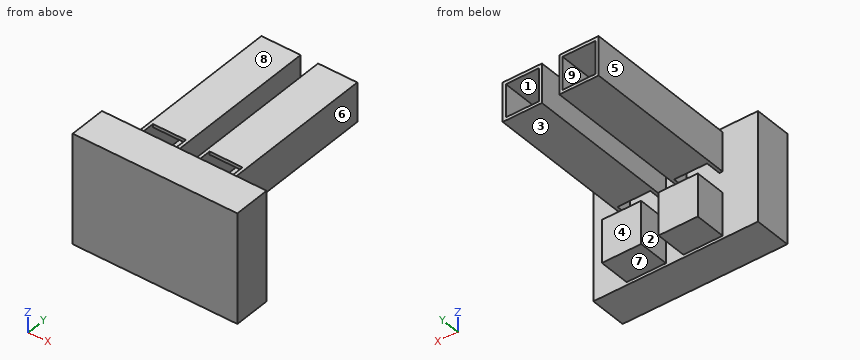
```python
from build123d import *

# Parameters (mm, degrees)
SKETCH1_W           = 266.7
SKETCH1_H           = 177.8
BOSS_EXTRUDE1_DEPTH = 59.944
SKETCH2_W           = 63.5
SKETCH2_H           = 63.5
SKETCH2_W_2         = 53.34
SKETCH2_H_2         = 53.34
BOSS_EXTRUDE2_DEPTH = 254
SKETCH3_W           = 53.34
SKETCH3_H           = 25.4
CUT_EXTRUDE1_DEPTH  = 254
SKETCH4_W           = 63.5
SKETCH4_H           = 69.373154479
BOSS_EXTRUDE3_DEPTH = 50.8
SKETCH5_R           = 6.35
CUT_EXTRUDE2_DEPTH  = 50.8


with BuildPart() as part:
    # Sketch1 → Boss-Extrude1 (new body)
    with BuildSketch(Plane(origin=(0, 0, 0), x_dir=(1, 0, 0), z_dir=(0, 1, 0))):
        with Locations((133.35, 88.9)):
            Rectangle(SKETCH1_W, SKETCH1_H)
    extrude(amount=BOSS_EXTRUDE1_DEPTH)

    # Sketch2 → Boss-Extrude2 (add)
    with BuildSketch(Plane(origin=(0, 59.944, 0), x_dir=(1, 0, 0), z_dir=(0, 1, 0))):
        with Locations((180.927983049, 38.1)):
            Rectangle(SKETCH2_W, SKETCH2_H)
        with Locations((180.927983049, 38.260329554)):
            Rectangle(SKETCH2_W_2, SKETCH2_H_2, mode=Mode.SUBTRACT)
        with Locations((89.140378802, 38.1)):
            Rectangle(SKETCH2_W, SKETCH2_H)
        with Locations((89.140378802, 38.260329554)):
            Rectangle(SKETCH2_W_2, SKETCH2_H_2, mode=Mode.SUBTRACT)
    extrude(amount=BOSS_EXTRUDE2_DEPTH)

    # Sketch3 → Cut-Extrude1 (cut)
    with BuildSketch(Plane.XY.offset(-6.35)):
        with Locations((89.140378802, 72.644)):
            Rectangle(SKETCH3_W, SKETCH3_H)
        with Locations((180.927983049, 72.644)):
            Rectangle(SKETCH3_W, SKETCH3_H)
    extrude(amount=-CUT_EXTRUDE1_DEPTH, mode=Mode.SUBTRACT)

    # Sketch4 → Boss-Extrude3 (add)
    with BuildSketch(Plane(origin=(0, 59.944, 0), x_dir=(1, 0, 0), z_dir=(0, 1, 0))):
        with Locations((89.140378802, 138.306511279)):
            Rectangle(SKETCH4_W, SKETCH4_H)
        with Locations((180.927983049, 138.306511279)):
            Rectangle(SKETCH4_W, SKETCH4_H)
    extrude(amount=BOSS_EXTRUDE3_DEPTH)

    # Sketch5 → Cut-Extrude2 (cut)
    with BuildSketch(Plane.XY.offset(-103.619934039)):
        with Locations((180.927983049, 72.644)):
            Circle(SKETCH5_R)
        with Locations((89.140378802, 72.644)):
            Circle(SKETCH5_R)
    extrude(amount=-CUT_EXTRUDE2_DEPTH, mode=Mode.SUBTRACT)


solid = part.part
```
Build history of the part. All positions in model axes, mm. Face numbers are marked on the shaded views. A direction names the side the tool comes from. Coordinates: 2 decimals unless noted, no trailing zeros. Order: outer loops, then holes, each group sorted by start corner. A loop starts at its lowest first (then second) coordinate and runs counter-clockwise, first axis right, second up. Notation, with made-up numbers: (-3.75, -15.5) -> (23.25, -15.5) arc R31 cw to (23.25, 22.5) -> close; hole circle Ø1 at (-22, -37). An arc over 180 degrees is marked (long way). Answer in a Markdown table with one row per item. Add a question column.
Q1. Band-saw the part on B-B, the plane x = 107. List the corners of the cut face in (y, z).
Q2. Band-saw the part on A-A, the plane y = 93.5. List the corners of the cut face in (x, z).
Q3. Wall check: line 1 along X through (y, z) = (98, -40); line 2 along Z through (x, y) = (202, 101.5); line 3 along Z through (x, y) = (172.5, 221). Give the ranges that are in metal, low to high. Write a range as [from, to].
Q4. Which spindle directions (+Z, -Z, +X, -X, +Y, -Y) get a long thin tool onto all of the face, cutting with end or side? Do the marked faces 1, 2, 3, 4 and 5. Say none if no direction does.
Q5. Drop flat-ended pins along their axis: pin 1 (10 mm diameter, centred on x = 180.93, y = 72.64, fed in from +Z); pin 2 (1 mm diameter, centred on x = 165, y = 110, fed in from -Z); pin 3 (19 mm diameter, centred on x = 173, z = -128, fed in from +Y). Give the stop position or say it passes through.
Q6. Band-saw the part on D-D, the plane z = -18. List the corners of the cut face in (x, y), then the cut area to 3 significant figures.
Q7. Mould opens along Z. For the marked faces 6, 7, 8 and 9 say: +Z half, -Z half, draft (parallel to the pull), parting line (faces both ways), or undercut.
Q8. Band-saw the part on C-C, the plane y = 221. List the corners of the cut face in (x, z), then the cut area to 3 significant figures.
Answers follow:
| question | item | result |
|---|---|---|
| 1 | outline | (0, -177.8) -> (59.94, -177.8) -> (59.94, -172.99) -> (110.74, -172.99) -> (110.74, -103.62) -> (59.94, -103.62) -> (59.94, 0) -> (0, 0) -> close; (85.34, -69.85) -> (313.94, -69.85) -> (313.94, -64.93) -> (85.34, -64.93) -> close; (85.34, -11.59) -> (313.94, -11.59) -> (313.94, -6.35) -> (85.34, -6.35) -> close |
| 2 | outline | (57.39, -172.99) -> (120.89, -172.99) -> (120.89, -103.62) -> (57.39, -103.62) -> close; (57.39, -69.85) -> (120.89, -69.85) -> (120.89, -6.35) -> (57.39, -6.35) -> close; (149.18, -172.99) -> (212.68, -172.99) -> (212.68, -103.62) -> (149.18, -103.62) -> close; (149.18, -69.85) -> (212.68, -69.85) -> (212.68, -6.35) -> (149.18, -6.35) -> close; hole (62.47, -64.93) -> (115.81, -64.93) -> (115.81, -11.59) -> (62.47, -11.59) -> close; hole (154.26, -64.93) -> (207.6, -64.93) -> (207.6, -11.59) -> (154.26, -11.59) -> close |
| 3 | line 1 | [57.39, 62.47], [115.81, 120.89], [149.18, 154.26], [207.6, 212.68] |
| 3 | line 2 | [-172.99, -103.62], [-69.85, -64.93], [-11.59, -6.35] |
| 3 | line 3 | [-69.85, -64.93], [-11.59, -6.35] |
| 4 | face 1 | +Y |
| 4 | face 2 | +Z, -Z, +Y |
| 4 | face 3 | +X, -X, +Y |
| 4 | face 4 | -Z, +X, -X, +Y |
| 4 | face 5 | +Z, -Z, -X, +Y |
| 5 | pin 1 | z = -154.42 |
| 5 | pin 2 | z = -172.99 |
| 5 | pin 3 | y = 110.74 |
| 6 | outline | (0, 0) -> (266.7, 0) -> (266.7, 59.94) -> (212.68, 59.94) -> (212.68, 313.94) -> (207.6, 313.94) -> (207.6, 59.94) -> (154.26, 59.94) -> (154.26, 313.94) -> (149.18, 313.94) -> (149.18, 59.94) -> (120.89, 59.94) -> (120.89, 313.94) -> (115.81, 313.94) -> (115.81, 59.94) -> (62.47, 59.94) -> (62.47, 313.94) -> (57.39, 313.94) -> (57.39, 59.94) -> (0, 59.94) -> close |
| 6 | area | 21,100 mm^2 |
| 7 | face 6 | draft |
| 7 | face 7 | -Z half |
| 7 | face 8 | +Z half |
| 7 | face 9 | undercut |
| 8 | outline | (57.39, -69.85) -> (120.89, -69.85) -> (120.89, -6.35) -> (57.39, -6.35) -> close; (149.18, -69.85) -> (212.68, -69.85) -> (212.68, -6.35) -> (149.18, -6.35) -> close; hole (62.47, -64.93) -> (115.81, -64.93) -> (115.81, -11.59) -> (62.47, -11.59) -> close; hole (154.26, -64.93) -> (207.6, -64.93) -> (207.6, -11.59) -> (154.26, -11.59) -> close |
| 8 | area | 2,370 mm^2 |
